```python
from build123d import *

# Parameters (mm, degrees)
BASE_FLANGE1_DEPTH      = 10
CUT_EXTRUDE1_DEPTH      = 22.737065119
CUT_EXTRUDE1_DEPTH_BACK = 22.737065119
SKETCH11_W              = 7
SKETCH11_H              = 5


# Sheet-metal steps are written as plain solids
with BuildPart() as part:
    # Sketch1 → Base-Flange1 (new, symmetric)
    with BuildSketch(Plane.XY):
        with BuildLine():
            Line((0, 0), (15, 0))
            ThreePointArc((15, 0), (16.147152873, 3.638304089), (13.120614758, 1.315959713))
            Line((13.120614758, 1.315959713), (11.711075827, 0.802929498))
            ThreePointArc((11.711075827, 0.802929498), (17.007517527, 4.867032155), (15, -1.5))
            Line((15, -1.5), (0, -1.5))
            Line((0, -1.5), (0, 0))
        make_face()
    extrude(amount=BASE_FLANGE1_DEPTH, both=True)

    # Sketch11 → Cut-Extrude1 (cut, two sides: drawn at the far end of the back side and taken through both)
    with BuildSketch(Plane(origin=(0, 0, 0), x_dir=(1, 0, 0), z_dir=(0, 1, 0)).offset(-CUT_EXTRUDE1_DEPTH_BACK)):
        with Locations((15, 7.5)):
            Rectangle(SKETCH11_W, SKETCH11_H)
        with Locations((15, -7.5)):
            Rectangle(SKETCH11_W, SKETCH11_H)
    extrude(amount=CUT_EXTRUDE1_DEPTH + CUT_EXTRUDE1_DEPTH_BACK, mode=Mode.SUBTRACT)


solid = part.part
```
Build history of the part. All positions in model axes, mm. A direction names the side the tool comes from. Round coordinates to 2 decimals unless told otherwise and drop trailing zeros. Order: outer loops, then holes, each group sorted by start corner. A loop starts at its lowest first (then second) coordinate and runs counter-clockwise, first axis right, second up. Notation, with made-up numbers: (81, 74.5) - (123, 74.5) arc R22 cw to (123, 105.5) - close; hole circle Ø1 at (43, -33). An arc over 180 degrees is marked (long way). Use a Markdown table: item, result.
1) Wall check: L1, parallel to X at y = 2, z = 2.75; L2, parallel to Y at x = 15, z = -0.25; L3, parallel to Y at x = 12, z = -1.5. Give the ranges that are in metal, low to high.
Recorded:
| item | result |
|---|---|
| L1 | x = 11.5 to 13, 17 to 18.5 |
| L2 | y = -1.5 to 0, 4 to 5.5 |
| L3 | y = -1.5 to 0, 0.91 to 3.8 |
2) Saw through at C-C on z = 7.25. Write the cut outline in (x, y), and give its area (4 significant figures).
Recorded:
| item | result |
|---|---|
| outline | (0, -1.5) - (11.5, -1.5) - (11.5, 0) - (0, 0) - close |
| area | 17.25 mm² |
3) Pull direction X, two halves, no side cores. Call faces 5 (the face through (16.2, 3.6, 0.1)), 6 (the face through (16.9, 4.94, 0.07)), 7 (the face through (6, -1, -10)): pulls with the +X half, pulls with the -X half, needs draft (parallel to the pull), parting line crosses it, or undercut.
Recorded:
| item | result |
|---|---|
| face 5 | undercut |
| face 6 | parting line crosses it |
| face 7 | needs draft |
4) Saw through at B-B on x = 12. Write the cut outline in (y, z), and give its area (3 significant figures).
Recorded:
| item | result |
|---|---|
| outline | (-1.5, -5) - (0, -5) - (0, 5) - (-1.5, 5) - close; (0.91, -5) - (3.8, -5) - (3.8, 5) - (0.91, 5) - close |
| area | 43.9 mm² |
5) Tool access for faces 1 (the face through (12.426, 1.063, 0.07)), 2 (the face through (11.5, -1, -7)), 3 (the face through (11.5, -1, 8)), 4 (the face through (7, 0, 0)): list every direction of +Z, -Z, +X, -X, +Y, -Y with a clear straight run to the whole face (end or side of a thin tool).
Recorded:
| item | result |
|---|---|
| face 1 | +Z, -Z |
| face 2 | -Z, +X, +Y, -Y |
| face 3 | +Z, +X, +Y, -Y |
| face 4 | +Z, -Z, -X |
6) Saw through at A-A on y = 2. Write the cut outline in (x, z).
Recorded:
| item | result |
|---|---|
| outline | (11.5, -5) - (13, -5) - (13, 5) - (11.5, 5) - close; (17, -5) - (18.5, -5) - (18.5, 5) - (17, 5) - close |
7) Saw through at D-D on x = 6.5. Write the cut outline in (y, z), and give its area (3 significant figures).
Recorded:
| item | result |
|---|---|
| outline | (-1.5, -10) - (0, -10) - (0, 10) - (-1.5, 10) - close |
| area | 30.0 mm² |
8) Flat gauge pins, fed straight in: pin 1 Ø10 at (x, z) = (14.5, -4.5) entering from +Y; pin 2 Ø1.2 at (y, z) = (-1, -7.5) entering from +X; pin 3 Ø2 at (y, z) = (0.5, 5.5) entering from +X; pin 4 Ø3.5 at (x, y) = (15.5, 1.5) entering from +Z. Where does each tip first touch, or does it go through?
Recorded:
| item | result |
|---|---|
| pin 1 | stops at y = 5.5 |
| pin 2 | stops at x = 11.5 |
| pin 3 | stops at x = 18.44 |
| pin 4 | stops at z = 5 |
